The drawing under review shows one solid part. Ordinate dimensions are in mm from its lowest x, y, z. Coordinates: 2 decimals unless noted, no trailing zeros. Loops run counter-clockwise (first coordinate to the right, second up) from the corner with the lowest first, then second, coordinate; pieces in that order, holes last. Notation, with made-up numbers: (73, 41.5) -> (103, 41.5) arc R19 ccw to (103, 49.5) -> close; hole circle Ø11 at (-22, 70). An arc over 180 degrees is marked (long way). Use a Markdown table: item, result.
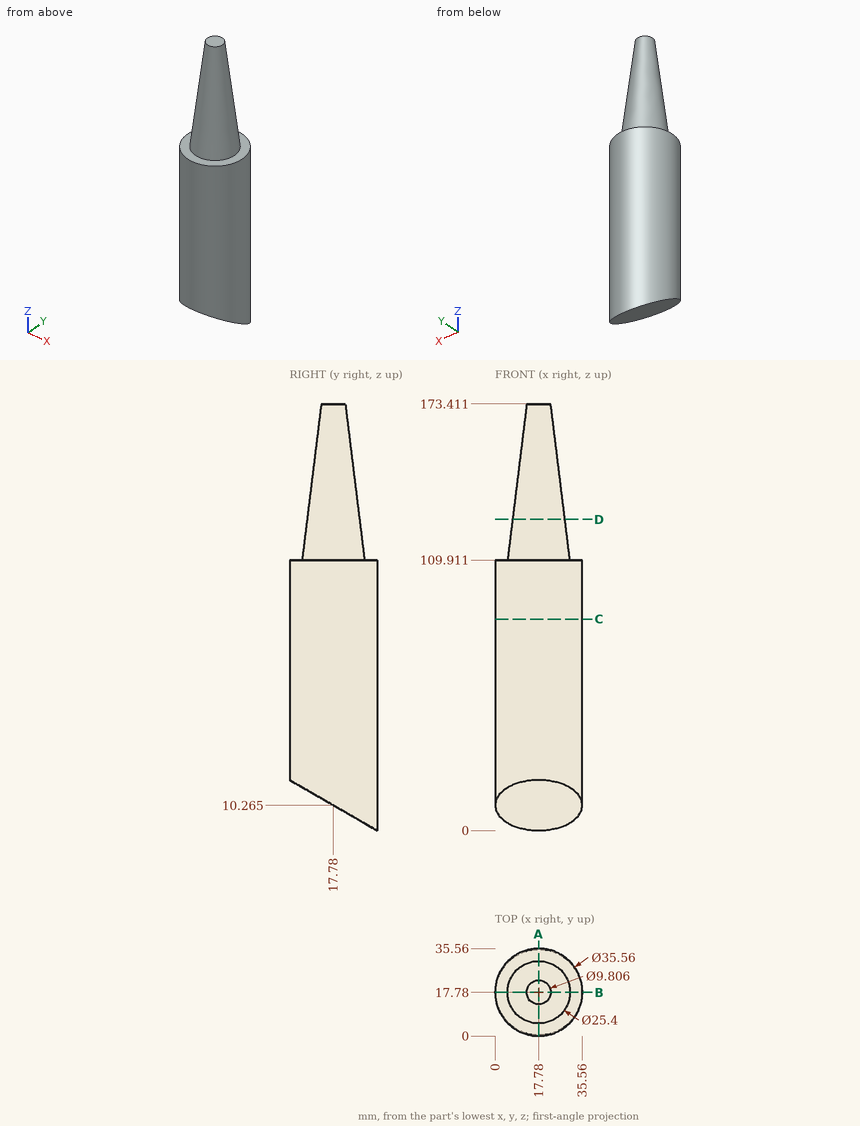
(1) For line 1 along Y through (x, z) = (24.5, 147.5) (1 decimal); line 2 along Z through (x, y) = (11, 32) (1 decimal); line 3 along Z through (x, y) = (17, 4.5), list the stretches that pass through material, from the lowest coordinate up.
Found:
| item | result |
|---|---|
| line 1 | y = 13.3 to 22.3 |
| line 2 | z = 2.1 to 109.9 |
| line 3 | z = 17.93 to 109.91 |
(2) Take a section at D-D on z = 126.5. Write out the cut boundary in (x, y), plus the area to 3 significant figures.
Found:
| item | result |
|---|---|
| outline | circle Ø21.33 at (17.78, 17.78) |
| area | 357 mm^2 |
(3) Take a section at B-B on y = 17.78. Write out the cut boundary in (x, z) (1 decimal).
Found:
| item | result |
|---|---|
| outline | (0, 10.3) -> (35.6, 10.3) -> (35.6, 109.9) -> (30.5, 109.9) -> (22.7, 173.4) -> (12.9, 173.4) -> (5.1, 109.9) -> (0, 109.9) -> close |
(4) Take a section at C-C on z = 86. Write out the cut boundary in (x, y).
Found:
| item | result |
|---|---|
| outline | circle Ø35.56 at (17.78, 17.78) |
(5) Take a section at A-A on x = 17.78. Write out the cut boundary in (y, z).
Found:
| item | result |
|---|---|
| outline | (0, 20.53) -> (35.56, 0) -> (35.56, 109.91) -> (30.48, 109.91) -> (22.68, 173.41) -> (12.88, 173.41) -> (5.08, 109.91) -> (0, 109.91) -> close |
(6) For pin 1 Ø5 at (x, y) = (4, 15) entering from -Z; pin 2 Ø5 at (y, z) = (6.5, 44) entering from +X; pin 3 Ø2 at (y, z) = (13, 32.5) entering from +X, all flat-tipped, find the tip position at first contact; note any pin that passes through.
Found:
| item | result |
|---|---|
| pin 1 | stops at z = 10.43 |
| pin 2 | stops at x = 33.24 |
| pin 3 | stops at x = 35.15 |
